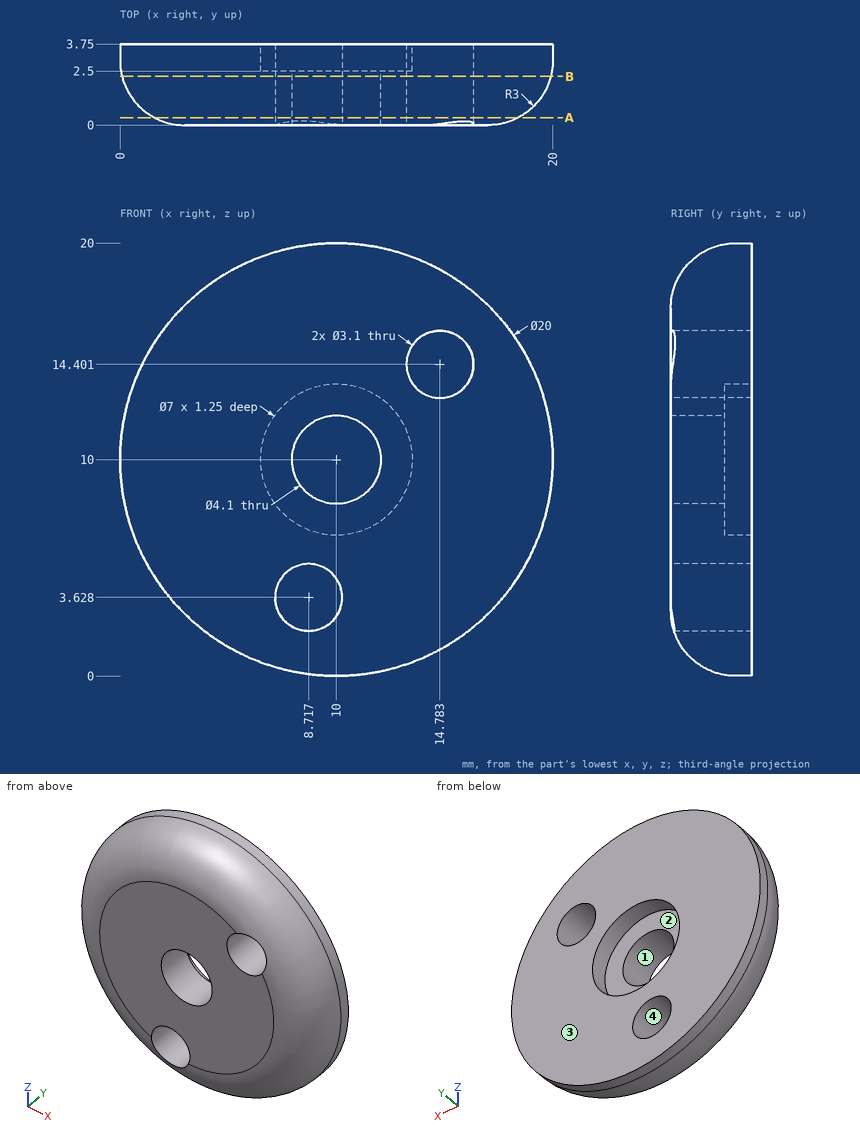
Design review of the part shown in the three views and the two pictorial views. Dimensions are in mm from the part's minimum x, y and z. A direction names the side the tool comes from. Round coordinates to 2 decimals unless told otherwise and drop trailing zeros. Loops run counter-clockwise (first coordinate to the right, second up) from the corner with the lowest first, then second, coordinate; pieces in that order, holes last. Notation, with made-up numbers: (-35, 26.5) -> (7, 26.5) arc R22 cw to (7, 48.5) -> close; hole circle Ø7 at (28, 65). An arc over 180 degrees is marked (long way). Use one line per item in the form item = value. Start each with the question number.
Q1. Machinability: for the marked faces 1 and 2, which of the approach directions +Z, -Z, +X, -X, +Y, -Y give a long, thin tool a straight path to every point of the face, cutting with its end or side? Answer none if there is none.
Q2. We need section B-B on y = 2.25. State how many separate pieces and enclosed holes the cut face has, then the cut area to 3 significant figures.
Q3. For pin 1 Ø1 at (y, z) = (3.5, 3) entering from -X; pin 2 Ø1.5 at (y, z) = (2, 15) entering from -X; pin 3 Ø2 at (y, z) = (1.5, 17.5) entering from -X, all flat-tipped, find the tip position at first contact; note any pin that passes through.
Q4. Wall thickness on line 1 along X through (y, z) = (0.6, 10); line 2 along X through (y, z) = (3.15, 3) (1 decimal); line 3 along Z through (x, y) = (15.5, 1.5) (1 decimal): over which ranges is each line inside the solid? List them lowest first. Write a range as [from, to].
Q5. Draft analysis for pull direction Z (two halves, no side actions). For the marked faces 3 and 4, state which applies: +Z half, -Z half, draft (parallel to the pull), parting line (faces both ways), or undercut.
Q6. We need section A-A on y = 0.35. Give the boundary of the cut face in (x, z), then the cut area to 3 significant figures.
Calculated:
q1.face_1 = +Y, -Y
q1.face_2 = +Y
q2.separate_pieces = 1
q2.enclosed_holes = 3
q2.area = 280 mm²
q3.pin_1 = 2.4
q3.pin_2 = 1.07
q3.pin_3 = 2.75
q4.line_1 = [1.2, 7.95], [12.05, 18.8]
q4.line_2 = [2.9, 7.3], [10.1, 17.1]
q4.line_3 = [2.1, 13], [15.8, 17.9]
q5.face_3 = draft
q5.face_4 = undercut
q6.outline = circle Ø16.81 at (10, 10); hole circle Ø3.1 at (8.72, 3.63); hole circle Ø4.1 at (10, 10); hole circle Ø3.1 at (14.78, 14.4)
q6.area = 194 mm²
